The listing builds one solid part. Answer for the finished solid, in the listing's coordinates (mm). Face numbers are marked on the shaded views. A direction names the side the tool comes from. Coordinates: 2 decimals unless noted, no trailing zeros. Order: outer loops, then holes, each group sorted by start corner. A loop starts at its lowest first (then second) coordinate and runs counter-clockwise, first axis right, second up. Notation, with made-up numbers: (33.5, -34) -> (43.5, -34) arc R23 ccw to (43.5, -12) -> close; hole circle Ø11 at (3.5, 83.25). An arc over 180 degrees is marked (long way). Answer in a Markdown table with one row per item.
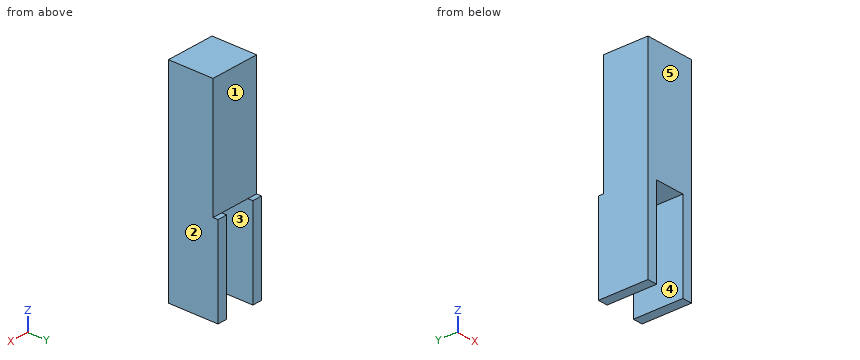
Autodesk Inventor part; units mm, degrees
ref_plane "YZ Plane" through (0, 0, 0) normal (1, 0, 0) x (0, 1, 0)
ref_plane "XZ Plane" through (0, 0, 0) normal (0, 1, 0) x (-1, 0, 0)
ref_plane "XY Plane" through (0, 0, 0) normal (0, 0, 1) x (1, 0, 0)
sketch "Sketch1" plane through (0, 0, 0) normal (0, 1, 0) x (-1, 0, 0)
  line L0 (0, 0) -> (0, -28.575)
  line L1 (0, 0) -> (15.875, 0)
  line L2 (15.875, 0) -> (15.875, -28.575)
  line L3 (0, -28.575) -> (15.875, -28.575)
  dimension "d0" = 28.575
  dimension "d1" = 15.875
extrude "Extrusion1" add sketch "Sketch1" along normal blind 22.225
sketch "Sketch2" plane through (-15.875, 0, 0) normal (0, 0, 1) x (1, 0, 0)
  line L0 (3.175, 3.175) -> (12.7, 3.175)
  line L1 (12.7, 3.175) -> (12.7, 19.05)
  line L2 (12.7, 19.05) -> (3.175, 19.05)
  line L3 (3.175, 19.05) -> (3.175, 3.175)
  line L4 (0, 0) -> (15.875, 0) construction
  line L5 (15.875, 0) -> (15.875, 22.225) construction
  line L6 (15.875, 22.225) -> (0, 22.225) construction
  line L7 (0, 22.225) -> (0, 0) construction
  dimension "d4" = 9.525
  dimension "d5" = 15.875
  dimension "d6" = 3.175
  dimension "d7" = 3.175
  dimension "d8" = 3.175
extrude "Extrusion2" cut sketch "Sketch2" against normal blind 50.8
sketch "Sketch3" plane through (-15.875, 0, 0) normal (0, 0, 1) x (1, 0, 0)
  line L0 (15.875, 0) -> (15.875, 22.225)
  line L1 (0, 22.225) -> (15.875, 22.225)
  line L2 (15.875, 22.225) -> (15.875, 19.05)
  line L3 (15.875, 19.05) -> (0, 19.05)
  line L4 (0, 19.05) -> (0, 22.225)
  line L5 (3.175, 19.05) -> (12.7, 19.05) construction
  line L6 (3.175, 19.05) -> (12.7, 19.05)
extrude "Extrusion3" cut sketch "Sketch3" against normal blind 50.8
sketch "Sketch4" plane through (-15.875, 0, 0) normal (0, 0, 1) x (1, 0, 0)
  line L0 (15.875, 0) -> (15.875, 19.05)
  line L1 (0, 0) -> (15.875, 0)
  line L2 (15.875, 0) -> (15.875, 3.175)
  line L3 (15.875, 3.175) -> (0, 3.175)
  line L4 (0, 3.175) -> (0, 0)
  point P0 (12.7, 3.175)
extrude "Extrusion4" cut sketch "Sketch4" against normal blind 50.8
sketch "Sketch5" plane through (-15.875, 19.05, 0) normal (0, 0, 1) x (1, 0, 0)
  line L0 (0, -15.875) -> (0, -1.5875)
  line L1 (0, -15.875) -> (3.175, -15.875)
  line L2 (0, -15.875) -> (3.175, -15.875)
  line L3 (3.175, -15.875) -> (3.175, -1.5875)
  line L4 (12.7, -15.875) -> (15.875, -15.875)
  line L5 (15.875, -15.875) -> (12.7, -15.875)
  line L6 (15.875, -15.875) -> (15.875, -1.5875)
  line L7 (12.7, -15.875) -> (12.7, -1.5875)
  line L8 (0, -1.5875) -> (3.175, -1.5875)
  line L9 (0, -15.875) -> (0, 0)
  line L10 (15.875, -1.5875) -> (12.7, -1.5875)
  line L11 (12.7, -15.875) -> (12.7, 0)
  line L12 (3.175, 0) -> (0, 0)
  line L13 (15.875, 0) -> (12.7, 0)
  line L14 (12.7, -15.875) -> (15.875, -15.875)
  line L15 (15.875, -15.875) -> (15.875, 0)
  point P0 (15.875, -19.05)
  dimension "d15" = 1.5875
  dimension "d16" = 1.5875
  dimension "d17" = 14.2875
extrude "Extrusion5" add sketch "Sketch5" along normal blind 6.35 contours L0 L8 L3 L1 | L7 L10 L6 L4
sketch "Sketch6" plane through (-3.175, 19.05, -28.575) normal (-1, 0, 0) x (0, 0, 1)
  line L0 (34.925, -15.875) -> (0, -15.875)
  line L1 (34.925, -1.5875) -> (28.575, -1.5875)
  line L2 (28.575, -1.5875) -> (28.575, -15.875)
  line L3 (28.575, -15.875) -> (34.925, -15.875)
  line L4 (34.925, -15.875) -> (34.925, -1.5875)
  point P0 (28.575, -19.05)
  dimension "d20" = 6.35
extrude "Extrusion6" add sketch "Sketch6" along normal blind 9.525
sketch "Sketch7" plane through (-15.875, 19.05, 6.35) normal (0, 0, 1) x (1, 0, 0)
  line L0 (0, -15.875) -> (15.875, -15.875)
  line L1 (15.875, -15.875) -> (15.875, -1.5875)
  line L2 (15.875, -1.5875) -> (0, -1.5875)
  line L3 (0, -1.5875) -> (0, -15.875)
  point P0 (15.875, -19.05)
extrude "Extrusion7" add sketch "Sketch7" along normal blind 31.75
properties part number "Limit Switch Container"
(1) A cutting plane is placed at A-A, the plane z = -17.5. Determine the outline of the cut face in (x, y) (3 decimals), then the cut area to 3 significant figures.
Check values:
| item | result |
|---|---|
| outline | (-15.875, 3.175) -> (-12.7, 3.175) -> (-12.7, 19.05) -> (-15.875, 19.05) -> close; (-3.175, 3.175) -> (0, 3.175) -> (0, 19.05) -> (-3.175, 19.05) -> close |
| area | 101 mm² |
(2) A cutting plane is placed at D-D, the plane z = 28.5. Determine the outline of the cut face in (x, y) (1 decimal), then the cut area to 3 significant figures.
Check values:
| item | result |
|---|---|
| outline | (-15.9, 3.2) -> (0, 3.2) -> (0, 17.5) -> (-15.9, 17.5) -> close |
| area | 227 mm² |
(3) A cutting plane is placed at C-C, the plane x = -6.5. Determine the outline of the cut face in (y, z) (1 decimal), then the cut area to 3 significant figures.
Check values:
| item | result |
|---|---|
| outline | (3.2, 0) -> (17.5, 0) -> (17.5, 38.1) -> (3.2, 38.1) -> close |
| area | 544 mm² |
(4) For a pull along X with two mould halves and no side action, classify the marked faces 1, 2 and 3 as released by +X, released by -X, zero draft, split by the parting line, or undercut.
Check values:
| item | result |
|---|---|
| face 1 | zero draft |
| face 2 | released by +X |
| face 3 | undercut |
(5) Which of the six approach directions +Z, -Z, +X, -X, +Y, -Y give full straight-line access (tool end or side, diameter ignored) to the marked faces 4 and 5?
Check values:
| item | result |
|---|---|
| face 4 | -Z, +Y, -Y |
| face 5 | +Z, -Z, +X, -X, -Y |
(6) Find the intervals of material crossed by line 1 along X through (y, z) = (15.25, -23.5) (3 decimals); line 2 along Z through (x, y) = (-7.25, 12.25); line 3 along Y through (x, z) = (-1.75, 32) (1 decimal), in increasing order. Write a range as from..to.
Check values:
| item | result |
|---|---|
| line 1 | -15.875..-12.7, -3.175..0 |
| line 2 | 0..38.1 |
| line 3 | 3.2..17.5 |
(7) Flat-ended cylindrical pins translate along their axes: pin 1 (1 mm diameter, centred on x = -10, y = 15.5, fed in from -Z); pin 2 (1.3 mm diameter, centred on x = -1.5, y = 18.5, fed in from +Z). Find the tip coordinate at first contact, or state that the pin passes through.
Check values:
| item | result |
|---|---|
| pin 1 | z = 0 |
| pin 2 | z = 0 |
(8) A cutting plane is placed at B-B, the plane y = 10.25. Determine the outline of the cut face in (x, z) (3 decimals).
Check values:
| item | result |
|---|---|
| outline | (-15.875, -28.575) -> (-12.7, -28.575) -> (-12.7, 0) -> (-3.175, 0) -> (-3.175, -28.575) -> (0, -28.575) -> (0, 38.1) -> (-15.875, 38.1) -> close |
